Could you check a few things on this model? Use its own coordinates, in mm. A direction names the side the tool comes from. Round coordinates to 2 decimals unless told otherwise and drop trailing zeros. Loops run counter-clockwise (first coordinate to the right, second up) from the corner with the lowest first, then second, coordinate; pieces in that order, holes last. Notation, with made-up numbers: (1, -21.75) -> (51, -21.75) arc R32 ccw to (51, 14.25) -> close; hole circle Ø1 at (20.25, 84.5). An arc over 180 degrees is marked (long way). One line per item, written item: value.
Autodesk Inventor part; units mm, degrees
ref_plane "YZ Plane" through (0, 0, 0) normal (1, 0, 0) x (0, 1, 0)
ref_plane "XZ Plane" through (0, 0, 0) normal (0, 1, 0) x (-1, 0, 0)
ref_plane "XY Plane" through (0, 0, 0) normal (0, 0, 1) x (1, 0, 0)
sketch "Sketch1" plane through (0, 0, 0) normal (0, 0, 1) x (1, 0, 0)
  line L0 (0, 0) -> (162, 0)
  line L1 (162, 0) -> (162, -300)
  line L2 (162, -300) -> (0, -300)
  line L3 (0, -300) -> (0, 0)
  dimension "d0" = 162
  dimension "d1" = 300
extrude "Extrusion1" add sketch "Sketch1" along normal blind 6
sketch "Sketch2" plane through (0, 0, 0) normal (0, 0, -1) x (-1, 0, 0)
  line L0 (0, 0) -> (-5.9, 0)
  line L1 (-5.9, 0) -> (-5.9, -22.5)
  line L2 (-5.9, -22.5) -> (0, -22.5)
  line L3 (0, -22.5) -> (0, 0)
  line L4 (-162, 0) -> (0, 0)
  line L5 (0, 0) -> (0, -300)
  line L6 (0, -37.5) -> (-5.9, -37.5)
  line L7 (-5.9, -37.5) -> (-5.9, -52.5)
  line L8 (-5.9, -52.5) -> (0, -52.5)
  line L9 (0, -52.5) -> (0, -37.5)
  line L10 (0, -30) -> (-5.9, -30)
  line L11 (0, -67.5) -> (-5.9, -67.5)
  line L12 (-5.9, -67.5) -> (-5.9, -82.5)
  line L13 (-5.9, -82.5) -> (0, -82.5)
  line L14 (0, -82.5) -> (0, -67.5)
  line L15 (0, -60) -> (-5.9, -60)
  line L16 (0, -97.5) -> (-5.9, -97.5)
  line L17 (-5.9, -97.5) -> (-5.9, -112.5)
  line L18 (-5.9, -112.5) -> (0, -112.5)
  line L19 (0, -112.5) -> (0, -97.5)
  line L20 (0, -90) -> (-5.9, -90)
  line L21 (0, -127.5) -> (-5.9, -127.5)
  line L22 (-5.9, -127.5) -> (-5.9, -142.5)
  line L23 (-5.9, -142.5) -> (0, -142.5)
  line L24 (0, -142.5) -> (0, -127.5)
  line L25 (0, -120) -> (-5.9, -120)
  line L26 (0, -157.5) -> (-5.9, -157.5)
  line L27 (-5.9, -157.5) -> (-5.9, -172.5)
  line L28 (-5.9, -172.5) -> (0, -172.5)
  line L29 (0, -172.5) -> (0, -157.5)
  line L30 (0, -150) -> (-5.9, -150)
  line L31 (0, -187.5) -> (-5.9, -187.5)
  line L32 (-5.9, -187.5) -> (-5.9, -202.5)
  line L33 (-5.9, -202.5) -> (0, -202.5)
  line L34 (0, -202.5) -> (0, -187.5)
  line L35 (0, -180) -> (-5.9, -180)
  line L36 (0, -217.5) -> (-5.9, -217.5)
  line L37 (-5.9, -217.5) -> (-5.9, -232.5)
  line L38 (-5.9, -232.5) -> (0, -232.5)
  line L39 (0, -232.5) -> (0, -217.5)
  line L40 (0, -210) -> (-5.9, -210)
  line L41 (0, -247.5) -> (-5.9, -247.5)
  line L42 (-5.9, -247.5) -> (-5.9, -262.5)
  line L43 (-5.9, -262.5) -> (0, -262.5)
  line L44 (0, -262.5) -> (0, -247.5)
  line L45 (0, -300) -> (-5.9, -300)
  line L46 (-5.9, -300) -> (-5.9, -277.5)
  line L47 (-5.9, -277.5) -> (0, -277.5)
  line L48 (0, -277.5) -> (0, -300)
  line L49 (-162, 0) -> (0, 0)
  line L50 (-81, 0) -> (-81, -60)
  line L51 (-162, 0) -> (-156.1, 0)
  line L52 (-156.1, 0) -> (-156.1, -22.5)
  line L53 (-156.1, -22.5) -> (-162, -22.5)
  line L54 (-162, -22.5) -> (-162, 0)
  line L55 (0, 0) -> (-162, 0)
  line L56 (-162, 0) -> (-162, -300)
  line L57 (-162, -37.5) -> (-156.1, -37.5)
  line L58 (-156.1, -37.5) -> (-156.1, -52.5)
  line L59 (-156.1, -52.5) -> (-162, -52.5)
  line L60 (-162, -52.5) -> (-162, -37.5)
  line L61 (-162, -30) -> (-156.1, -30)
  line L62 (-162, -67.5) -> (-156.1, -67.5)
  line L63 (-156.1, -67.5) -> (-156.1, -82.5)
  line L64 (-156.1, -82.5) -> (-162, -82.5)
  line L65 (-162, -82.5) -> (-162, -67.5)
  line L66 (-162, -60) -> (-156.1, -60)
  line L67 (-162, -97.5) -> (-156.1, -97.5)
  line L68 (-156.1, -97.5) -> (-156.1, -112.5)
  line L69 (-156.1, -112.5) -> (-162, -112.5)
  line L70 (-162, -112.5) -> (-162, -97.5)
  line L71 (-162, -90) -> (-156.1, -90)
  line L72 (-162, -127.5) -> (-156.1, -127.5)
  line L73 (-156.1, -127.5) -> (-156.1, -142.5)
  line L74 (-156.1, -142.5) -> (-162, -142.5)
  line L75 (-162, -142.5) -> (-162, -127.5)
  line L76 (-162, -120) -> (-156.1, -120)
  line L77 (-162, -157.5) -> (-156.1, -157.5)
  line L78 (-156.1, -157.5) -> (-156.1, -172.5)
  line L79 (-156.1, -172.5) -> (-162, -172.5)
  line L80 (-162, -172.5) -> (-162, -157.5)
  line L81 (-162, -150) -> (-156.1, -150)
  line L82 (-162, -187.5) -> (-156.1, -187.5)
  line L83 (-156.1, -187.5) -> (-156.1, -202.5)
  line L84 (-156.1, -202.5) -> (-162, -202.5)
  line L85 (-162, -202.5) -> (-162, -187.5)
  line L86 (-162, -180) -> (-156.1, -180)
  line L87 (-162, -217.5) -> (-156.1, -217.5)
  line L88 (-156.1, -217.5) -> (-156.1, -232.5)
  line L89 (-156.1, -232.5) -> (-162, -232.5)
  line L90 (-162, -232.5) -> (-162, -217.5)
  line L91 (-162, -210) -> (-156.1, -210)
  line L92 (-162, -247.5) -> (-156.1, -247.5)
  line L93 (-156.1, -247.5) -> (-156.1, -262.5)
  line L94 (-156.1, -262.5) -> (-162, -262.5)
  line L95 (-162, -262.5) -> (-162, -247.5)
  line L96 (-162, -300) -> (-156.1, -300)
  line L97 (-156.1, -300) -> (-156.1, -277.5)
  line L98 (-156.1, -277.5) -> (-162, -277.5)
  line L99 (-162, -277.5) -> (-162, -300)
  line L100 (0, 0) -> (-162, 0)
  point P0 (-162, -277.5)
  point P1 (0, -277.5)
  point P2 (0, -262.5)
  point P3 (0, -232.5)
  point P4 (0, -202.5)
  point P5 (-162, -82.5)
  point P6 (0, -172.5)
  point P7 (-162, -157.5)
  point P8 (0, -142.5)
  point P9 (-162, -142.5)
  point P10 (0, -112.5)
  point P11 (-162, -97.5)
  point P12 (0, -82.5)
  point P13 (-162, -247.5)
  point P14 (-156.1, 0)
  point P15 (-162, -232.5)
  dimension "d4" = 0
  dimension "d5" = 5.9
  dimension "d6" = 0
  dimension "d7" = 22.5
  dimension "d8" = 5.9
  dimension "d9" = 15
  dimension "d10" = 15
  dimension "d13" = 30
  dimension "d18" = 22.5
  dimension "d19" = 5.9
extrude "Extrusion2" cut sketch "Sketch2" against normal mid plane 24
sketch "Sketch3" plane through (0, 0, 6) normal (0, 0, 1) x (1, 0, 0)
  circle A0 centre (28.4, -30) radius 2.5
  circle A1 centre (133.4, -30) radius 2.5
  circle A2 centre (28.4, -135) radius 2.5
  circle A3 centre (133.4, -135) radius 2.5
  circle A4 centre (28.4, -165) radius 2.5
  circle A5 centre (133.4, -165) radius 2.5
  circle A6 centre (28.4, -270) radius 2.5
  circle A7 centre (133.4, -270) radius 2.5
  line L0 (5.9, 0) -> (5.9, -22.5)
  line L1 (156.1, -22.5) -> (156.1, 0)
  line L2 (5.9, -300) -> (156.1, -300)
  line L3 (156.1, 0) -> (5.9, 0)
  circle A8 centre (81, -82.5) radius 56.9012
  circle A9 centre (81, -217.5) radius 58.271
  line L4 (156.1, -202.5) -> (156.1, -187.5)
  point P0 (0, 0)
  dimension "d22" = 5
  dimension "d23" = 5
  dimension "d24" = 5
  dimension "d25" = 5
  dimension "d26" = 5
  dimension "d27" = 5
  dimension "d28" = 5
  dimension "d29" = 5
  dimension "d30" = 105
  dimension "d31" = 105
  dimension "d32" = 105
  dimension "d33" = 22.5
  dimension "d34" = 150.2
  dimension "d35" = 105
  dimension "d36" = 105
  dimension "d37" = 105
  dimension "d38" = 30
  dimension "d39" = 22.5
  dimension "d40" = 30
  dimension "d41" = 105
  dimension "d44" = 135
  dimension "d45" = 30
  dimension "d46" = 82.5
  dimension "d47" = 75.1
  dimension "d48" = 75.1
extrude "Extrusion3" cut sketch "Sketch3" along normal mid plane 24
equation "\"d2\" = WoodWidth"
equation "\"d5\" = WoodWidth - LaserWith"
equation "\"d8\" = d5"
equation "\"d18\" = d7"
equation "\"d19\" = d5"
equation "\"d20\" = 4 * WoodWidth"
equation "\"d39\" = d33"
equation "\"d40\" = d38"
equation "\"d42\" = 4 * WoodWidth"
equation "\"WoodWidth\" = 6"
equation "\"LaserWith\" = 0.1"
properties part number "BackFrontPannel"
(1) If we section it at D-D, the plane z = 1.9: Give the number of separate pieces and of enclosed holes in the cut face, then the cut area to 3 significant figures.
Recorded:
separate pieces: 1
enclosed holes: 10
area: 25,700 mm²
(2) If we section it at B-B, the plane y = -122: Please give me the cut outline in (x, z), then the cut area to 3 significant figures.
Recorded:
outline: (0, 0) -> (40.04, 0) -> (40.04, 6) -> (0, 6) -> close; (121.96, 0) -> (162, 0) -> (162, 6) -> (121.96, 6) -> close
area: 481 mm²
(3) Thinking about a two-plate mould opening in Y: for faces 1 (the face through (162, -210, 3)), 2 (the face through (3, -202.5, 3)), 3 (the face through (3, -22.5, 3)), 4 (the face through (3, -277.5, 3)), which applies, released by +Y, released by -Y, zero draft, split by the parting line, or undercut?
Recorded:
face 1: zero draft
face 2: undercut
face 3: released by +Y
face 4: released by -Y
(4) If I drill on L1, parallel to Y at x = 78.5, z = 2.3; L2, parallel to Y at x = 81, z = 4.2; L3, parallel to X at y = -165, z = 1.6, over which ranges is the centre line in solid material (lowest first)?
Recorded:
L1: -300 to -275.72, -159.28 to -139.35, -25.65 to 0
L2: -300 to -275.77, -159.23 to -139.4, -25.6 to 0
L3: 5.9 to 25.9, 30.9 to 55.72, 106.28 to 130.9, 135.9 to 156.1
(5) For faces 5 (the face through (5.9, -165, 3)), 6 (the face through (156.1, -289, 3)), 7 (the face through (156.1, -135, 3)), which set-ups out of +Z, -Z, +X, -X, +Y, -Y let a thin tool reach every point of the face, with its end or its side?
Recorded:
face 5: +Z, -Z, -X
face 6: +Z, -Z, +X, -Y
face 7: +Z, -Z, +X
(6) I'm going to push flat-ended pins straight in: pin 1 Ø1.8 at (x, z) = (4, 3.5) entering from -Y; pin 2 Ø3 at (y, z) = (-165.5, 4.5) entering from -X; pin 3 Ø3 at (x, z) = (3, 1.5) entering from +Y. Where does each tip first touch, or does it pass through?
Recorded:
pin 1: y = -277.5
pin 2: x = 5.9
pin 3: y = -22.5
(7) If we section it at A-A, the plane x = 81: Please give me the cut outline in (y, z).
Recorded:
outline: (-300, 0) -> (-275.77, 0) -> (-275.77, 6) -> (-300, 6) -> close; (-159.23, 0) -> (-139.4, 0) -> (-139.4, 6) -> (-159.23, 6) -> close; (-25.6, 0) -> (0, 0) -> (0, 6) -> (-25.6, 6) -> close
(8) If we section it at C-C, the plane x = 113.5: Please give me the cut outline in (y, z).
Recorded:
outline: (-300, 0) -> (-265.87, 0) -> (-265.87, 6) -> (-300, 6) -> close; (-169.13, 0) -> (-129.21, 0) -> (-129.21, 6) -> (-169.13, 6) -> close; (-35.79, 0) -> (0, 0) -> (0, 6) -> (-35.79, 6) -> close
